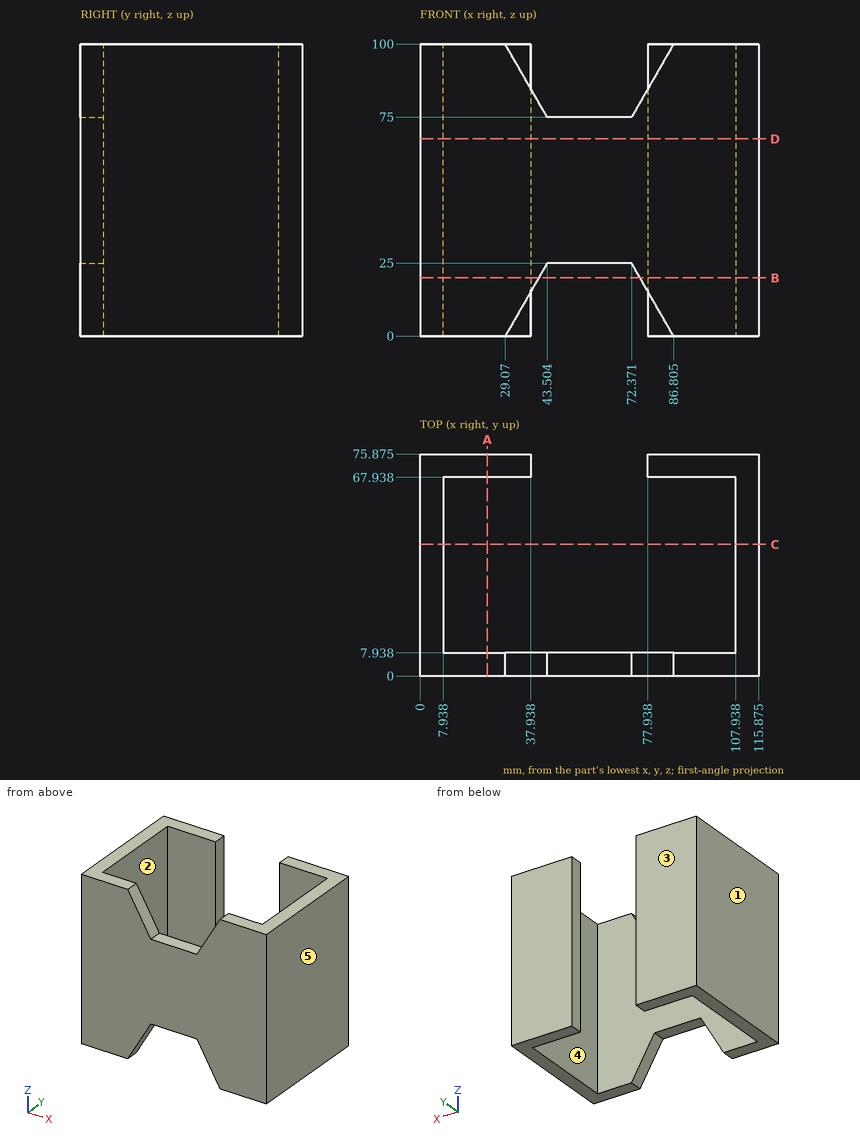
Geometry check sheet. Reference: drawing and pictorial views, mm from the part's lowest x, y, z. A direction names the side the tool comes from. Give positions to 0.01 mm unless a question says otherwise; leave off trailing zeros. Order: outer loops, then holes, each group sorted by start corner. A loop starts at its lowest first (then second) coordinate and runs counter-clockwise, first axis right, second up. Notation, with made-up numbers: M 33.5,1.5 L 82.5,1.5 A32 cw 82.5,30.5 Z; hole C 52.5,33 d11. An arc over 180 degrees is marked long. Answer in a Markdown table with one row per item.
1) Cross-section at B-B, the plane z = 20. Enter the section's corners in (x, y) (1 decimal), plus the area to 3 significant figures.
Filled sheet:
| item | result |
|---|---|
| outline | M 0,0 L 40.6,0 L 40.6,7.9 L 7.9,7.9 L 7.9,67.9 L 37.9,67.9 L 37.9,75.9 L 0,75.9 Z; M 75.3,0 L 115.9,0 L 115.9,75.9 L 77.9,75.9 L 77.9,67.9 L 107.9,67.9 L 107.9,7.9 L 75.3,7.9 Z |
| area | 2,200 mm2 |
2) Cross-section at A-A, the plane x = 23. Enter the section's corners in (y, z) (1 decimal), plus the area to 3 significant figures.
Filled sheet:
| item | result |
|---|---|
| outline | M 0,0 L 7.9,0 L 7.9,100 L 0,100 Z; M 67.9,0 L 75.9,0 L 75.9,100 L 67.9,100 Z |
| area | 1,590 mm2 |
3) Release check for a two-part mould opening along X. For the marked faces 1, 2 and 3 record: +X half, -X half, draft (parallel to the pull), parting line (faces both ways), or undercut.
Filled sheet:
| item | result |
|---|---|
| face 1 | -X half |
| face 2 | undercut |
| face 3 | draft |
4) Cross-section at C-C, the plane y = 45. Enter the section's corners in (x, z) (1 decimal), plus the area to 3 significant figures.
Filled sheet:
| item | result |
|---|---|
| outline | M 0,0 L 7.9,0 L 7.9,100 L 0,100 Z; M 107.9,0 L 115.9,0 L 115.9,100 L 107.9,100 Z |
| area | 1,590 mm2 |
5) Access from +Z, -Z, +X, -X, +Y, -Y to the whole of each face (thin tool, end or side, straight path). Record for the marked faces 4 and 5.
Filled sheet:
| item | result |
|---|---|
| face 4 | +Z, -Z |
| face 5 | +Z, -Z, +X, +Y, -Y |
6) Cross-section at D-D, the plane z = 67.5. Enter the section's corners in (x, y) (1 decimal).
Filled sheet:
| item | result |
|---|---|
| outline | M 0,0 L 115.9,0 L 115.9,75.9 L 77.9,75.9 L 77.9,67.9 L 107.9,67.9 L 107.9,7.9 L 7.9,7.9 L 7.9,67.9 L 37.9,67.9 L 37.9,75.9 L 0,75.9 Z |
7) Gauge pin test, flat ends, axial feed: P1, Ø10, axis at x = 102.5, y = 19.5, coming from the -Z side; P2, Ø6.5, axis at x = 64.5, y = 5.5, coming from the -Z side; P3, Ø2.5, axis at x = 57.5, y = 5.5, coming from the +Z side. Record the tip position at first contact, or that the pin passes through.
Filled sheet:
| item | result |
|---|---|
| P1 | passes through |
| P2 | stops at z = 25 |
| P3 | stops at z = 75 |
8) Thickness scan on L1, parallel to X at y = 18, z = 89 (1 decimal); L2, parallel to X at y = 70, z = 78.5 (1 decimal); L3, parallel to Y at x = 34, z = 14 (1 decimal). Record the ranges inside material, lowest first. Write a range as [from, to].
Filled sheet:
| item | result |
|---|---|
| L1 | x = [0, 7.9], [107.9, 115.9] |
| L2 | x = [0, 37.9], [77.9, 115.9] |
| L3 | y = [0, 7.9], [67.9, 75.9] |
